Design review of the part built by this model. Coordinates are the model's own, in mm. A direction names the side the tool comes from. Give positions to 0.01 mm unless a question says otherwise; leave off trailing zeros. Loops run counter-clockwise (first coordinate to the right, second up) from the corner with the lowest first, then second, coordinate; pieces in that order, holes last. Notation, with made-up numbers: (47, 57.5) -> (86, 57.5) arc R30 cw to (86, 95.5) -> close; hole circle Ø1 at (73, 89.5). An arc over 180 degrees is marked (long way). Use CSV: the item, a comma, the result in double quotes. Start each with the question number.
Item 1: We need section A-A (z = 2). State the section outline as (x, y) points, plus the area to 3 significant figures.
Item 2: We need section D-D (x = 3.25). State the section outline as (y, z) points.
Item 3: Clearance check with a flat-ended pin moving along its axis: pin 1 (1.7 mm diameter, centred on y = 0.5, z = 2.5, fed in from +X). State where the tip first meets the part, or that it passes through.
Item 4: We need section C-C (z = 0.75). State the section outline as (x, y) points.
Item 5: We need section B-B (x = -4). State the section outline as (y, z) points.
Item 6: For faces 4 (the face through (2, 1.675, 2)), 5 (the face through (-10, 0, 2)), 6 (the face through (-10, -1, 2)), list the 3-axis set-ups (+Z, -Z, +X, -X, +Y, -Y) from which the entire face can be reached by the end or side of a thin tool; tool diameter is ignored.
Item 7: The part is to be moulded in two halves that separate along X. For faces 1 (the face through (-5, -0.5, 0)), 2 (the face through (0, 2, 2)), 3 (the face through (2.502, 2.357, 1.392)), say which applies: +X half, -X half, draft (parallel to the pull), parting line (faces both ways), or undercut.
Item 8: Wall thickness on line 1 along X through (y, z) = (-0.7, 2.3); line 2 along Z through (x, y) = (-2.75, -0.75); line 3 along Y through (x, z) = (1.5, 1.5): over which ranges is each line inside the solid? List them lowest first. Write a range as from..to.
from build123d import *

# Parameters (mm, degrees)
F0_W     = 20
F0_H     = 4
F1_DEPTH = 1
F2_W     = 3.0585520435
F2_H     = 4
F2_W_2   = 1
F3_DEPTH = 1
F4_W     = 1.3837967999
F4_H     = 4
F5_DEPTH = 4
F6_R     = 1
F7_DEPTH = 2
F8_F1_R  = 0.3
F8_F2_R  = 0.3


with BuildPart() as f1:
    # F0 (on Front) → F1 (new body)
    with BuildSketch(Plane.XZ):
        with Locations((-10, 2)):
            Rectangle(F0_W, F0_H)
    extrude(amount=F1_DEPTH)

    # F2 (on face) → F3 (join)
    with BuildSketch(Plane.YZ):
        with Locations((1.5292760218, 2)):
            Rectangle(F2_W, F2_H)
        with Locations((-0.5, 2)):
            Rectangle(F2_W_2, F2_H)
    extrude(amount=F3_DEPTH)

    # F4 (on face) → F5 (join)
    with BuildSketch(Plane.YZ.offset(1)):
        with Locations((2.3666536435, 2)):
            Rectangle(F4_W, F4_H)
    extrude(amount=F5_DEPTH)

    # F6 (on face) → F7 (cut)
    with BuildSketch(Plane.XZ.offset(-1.6747552436)):
        with Locations((3.2954369672, 2)):
            Circle(F6_R)
    extrude(amount=-F7_DEPTH, mode=Mode.SUBTRACT)

    # F8: fillet of radius 0.3 on 18 edges, made by hand

    # F8_f1
    f8_f1_edges = [f1.edges().sort_by_distance(p)[0] for p in [
        (0, 0, 2),
        (1, 1.6747552436, 2),
    ]]
    fillet(f8_f1_edges, radius=F8_F1_R)

    # F8_f2
    f8_f2_edges = [f1.edges().sort_by_distance(p)[0] for p in [
        (-9.5, -1, 0),
        (1, -1, 2),
        (-9.5, -1, 4),
        (-20, -1, 2),
        (-10.15, 0, 0),
        (-10.15, 0, 4),
        (-20, 0, 2),
        (2.5, 3.0585520435, 0),
        (2.5, 3.0585520435, 4),
        (5, 3.0585520435, 2),
        (0, 3.0585520435, 2),
        (5, 1.6747552436, 2),
        (5, 2.3666536435, 0),
        (5, 2.3666536435, 4),
        (3.15, 1.6747552436, 0),
        (3.15, 1.6747552436, 4),
        (1.0878679656, 1.5868872779, 4),
        (1.0878679656, 1.5868872779, 0),
        (-0.0878679656, 0.0878679656, 4),
        (-0.0878679656, 0.0878679656, 0),
    ]]
    fillet(f8_f2_edges, radius=F8_F2_R)


solid = f1.part
Results found:
1,outline,"(-20, -0.7) arc R0.3 ccw to (-19.7, -1) -> (0.7, -1) arc R0.3 ccw to (1, -0.7) -> (1, 1.37) arc R0.3 cw to (1.3, 1.67) -> (2.3, 1.67) -> (2.3, 3.06) -> (0.3, 3.06) arc R0.3 ccw to (0, 2.76) -> (0, 0.3) arc R0.3 cw to (-0.3, 0) -> (-19.7, 0) arc R0.3 ccw to (-20, -0.3) -> close; (4.3, 1.67) -> (4.7, 1.67) arc R0.3 ccw to (5, 1.97) -> (5, 2.76) arc R0.3 ccw to (4.7, 3.06) -> (4.3, 3.06) -> close"
1,area,"26.7 mm²"
2,outline,"(1.67, 0.3) arc R0.3 ccw to (1.97, 0) -> (2.76, 0) arc R0.3 ccw to (3.06, 0.3) -> (3.06, 1) -> (1.67, 1) -> close; (1.67, 3) -> (3.06, 3) -> (3.06, 3.7) arc R0.3 ccw to (2.76, 4) -> (1.97, 4) arc R0.3 ccw to (1.67, 3.7) -> close"
3,pin 1,"x = 1"
4,outline,"(-20, -0.7) arc R0.3 ccw to (-19.7, -1) -> (0.7, -1) arc R0.3 ccw to (1, -0.7) -> (1, 1.37) arc R0.3 cw to (1.3, 1.67) -> (4.7, 1.67) arc R0.3 ccw to (5, 1.97) -> (5, 2.76) arc R0.3 ccw to (4.7, 3.06) -> (0.3, 3.06) arc R0.3 ccw to (0, 2.76) -> (0, 0.3) arc R0.3 cw to (-0.3, 0) -> (-19.7, 0) arc R0.3 ccw to (-20, -0.3) -> close"
5,outline,"(-1, 0.3) arc R0.3 ccw to (-0.7, 0) -> (-0.3, 0) arc R0.3 ccw to (0, 0.3) -> (0, 3.7) arc R0.3 ccw to (-0.3, 4) -> (-0.7, 4) arc R0.3 ccw to (-1, 3.7) -> close"
6,face 4,"+Z, -Z, +X, -Y"
6,face 5,"+Z, -Z, -X, +Y"
6,face 6,"+Z, -Z, +X, -X, -Y"
7,face 1,"draft"
7,face 2,"-X half"
7,face 3,"undercut"
8,line 1,"-20..1"
8,line 2,"0..4"
8,line 3,"1.67..3.06"
